Geometry: final body of the model. Coordinates: model frame, mm. A direction names the side the tool comes from. Give positions to 0.01 mm unless a question says otherwise; leave off trailing zeros. Write each loop counter-clockwise with the first axis right and the second up, starting at its lowest first coordinate (ties: lowest second). Pieces come first, ordered by that corner, then holes.
from build123d import *

# Parameters (mm, degrees)
SKETCH1_W                = 80
SKETCH1_H                = 80
BOSS_EXTRUDE1_DEPTH      = 2
SKETCH2_W                = 80
SKETCH2_H                = 2
BOSS_EXTRUDE2_DEPTH      = 50
SKETCH3_W                = 2
SKETCH3_H                = 76
BOSS_EXTRUDE3_DEPTH      = 50
CUT_EXTRUDE2_DEPTH       = 100
SKETCH6_W                = 2
SKETCH6_H                = 76
BOSS_EXTRUDE4_DEPTH      = 16.666666667
BOSS_EXTRUDE5_DEPTH      = 2
BOSS_EXTRUDE5_DEPTH_BACK = 82
SKETCH7_W                = 84
SKETCH7_H                = 9.392000317
SKETCH8_W                = 14
SKETCH8_H                = 80
CUT_EXTRUDE3_DEPTH       = 50


with BuildPart() as part:
    # Sketch1 → Boss-Extrude1 (new body)
    with BuildSketch(Plane.XY):
        with Locations((40, 40)):
            Rectangle(SKETCH1_W, SKETCH1_H)
    extrude(amount=BOSS_EXTRUDE1_DEPTH)

    # Sketch2 → Boss-Extrude2 (add)
    with BuildSketch(Plane(origin=(0, 0, 0), x_dir=(-1, 0, 0), z_dir=(0, 0, -1))):
        with Locations((-40, 79)):
            Rectangle(SKETCH2_W, SKETCH2_H)
        with Locations((-40, 1)):
            Rectangle(SKETCH2_W, SKETCH2_H)
    extrude(amount=BOSS_EXTRUDE2_DEPTH)

    # Sketch3 → Boss-Extrude3 (add)
    with BuildSketch(Plane(origin=(0, 0, 0), x_dir=(-1, 0, 0), z_dir=(0, 0, -1))):
        with Locations((-79, 40)):
            Rectangle(SKETCH3_W, SKETCH3_H)
    extrude(amount=BOSS_EXTRUDE3_DEPTH)

    # Sketch5 → Cut-Extrude2 (cut)
    with BuildSketch(Plane(origin=(0, 80, 0), x_dir=(1, 0, 0), z_dir=(0, 1, 0))):
        Polygon((80, 50), (0, 16.666666667), (0, 50), align=None)
    extrude(amount=-CUT_EXTRUDE2_DEPTH, mode=Mode.SUBTRACT)

    # Sketch6 → Boss-Extrude4 (add)
    with BuildSketch(Plane(origin=(0, 0, 0), x_dir=(-1, 0, 0), z_dir=(0, 0, -1))):
        with Locations((-1, 40)):
            Rectangle(SKETCH6_W, SKETCH6_H)
    extrude(amount=BOSS_EXTRUDE4_DEPTH)

    # Sketch7 → Boss-Extrude5 (add, two sides: drawn at the far end of the back side and taken through both)
    with BuildSketch(Plane(origin=(0, 80, 0), x_dir=(1, 0, 0), z_dir=(0, 1, 0)).offset(-BOSS_EXTRUDE5_DEPTH_BACK)):
        with Locations((52, 7.482577596)):
            Rectangle(SKETCH7_W, SKETCH7_H)
    extrude(amount=BOSS_EXTRUDE5_DEPTH + BOSS_EXTRUDE5_DEPTH_BACK)

    # Sketch8 → Cut-Extrude3 (cut)
    with BuildSketch(Plane.XY.offset(-2.786577437)):
        with Locations((87, 40)):
            Rectangle(SKETCH8_W, SKETCH8_H)
    extrude(amount=-CUT_EXTRUDE3_DEPTH, mode=Mode.SUBTRACT)


solid = part.part
Q1. Section C-C on y = 35. Output: boundary loops of the cut face in (x, z), plus the area to 3 significant figures.
Filled sheet:
outline: (0, -16.67) - (2, -16.67) - (2, 0) - (78, 0) - (78, -2.79) - (10, -2.79) - (10, -12.18) - (78, -12.18) - (78, -49.17) - (80, -50) - (80, 2) - (0, 2) - close
area: 931 mm2
Q2. Section D-D on x = 58. Output: boundary loops of the cut face in (y, z).
Filled sheet:
outline: (-2, -12.18) - (0, -12.18) - (0, -40.83) - (2, -40.83) - (2, -12.18) - (78, -12.18) - (78, -40.83) - (80, -40.83) - (80, -12.18) - (82, -12.18) - (82, -2.79) - (80, -2.79) - (80, 2) - (0, 2) - (0, -2.79) - (-2, -2.79) - close; hole (2, -2.79) - (78, -2.79) - (78, 0) - (2, 0) - close
Q3. Pull-direction query (X, two-part tool) for faces 5 (the flat face through (80, 39, -24)), 6 (the flat face through (39, 41, 0)), 7 (the flat face through (0, 39, -7)), 8 (the flat face through (39, 41, 2)); classes: released by +X, released by -X, zero draft, split by the parting line, or undercut.
Filled sheet:
face 5: released by +X
face 6: undercut
face 7: released by -X
face 8: zero draft
Q4. Section B-B on z = -43. Output: boundary loops of the cut face in (x, y).
Filled sheet:
outline: (63.2, 0) - (80, 0) - (80, 80) - (63.2, 80) - (63.2, 78) - (78, 78) - (78, 2) - (63.2, 2) - close
Q5. Section A-A on x = 88. Output: boundary loops of the cut face in (y, z).
Filled sheet:
outline: (-2, -12.18) - (0, -12.18) - (0, -2.79) - (-2, -2.79) - close; (80, -12.18) - (82, -12.18) - (82, -2.79) - (80, -2.79) - close
Q6. Pin query (flat end, axial travel): P1, Ø0.6, axis at x = 65, y = -1.5, coming from the +Z side; P2, Ø10, axis at y = 23, z = -24.5, coming from the +X side; P3, Ø10, axis at x = 54.5, z = -30.5, coming from the -Y side. Return the tip coordinate at first contact, or that it passes through.
Filled sheet:
P1: stops at z = -2.79
P2: stops at x = 80
P3: stops at y = 0
Q7. Ray query, line 1 along X through (y, z) = (56, -13); line 2 along Z through (x, y) = (61, 36). Return the intervals inside material, ascending.
Filled sheet:
line 1: x = 0 to 2, 78 to 80
line 2: z = -12.18 to -2.79, 0 to 2
Q8. Access query for faces 1 (the flat face through (87, 0, -7)), 2 (the flat face through (48, 78, -19)), 3 (the flat face through (51, -2, -8)), 4 (the flat face through (10, 39, -7)). Directions: +Z, -Z, +X, -X, +Y, -Y. A direction counts if a zero-diameter tool reaches every point of the face in a straight line with its end or side. Return the directions, or none.
Filled sheet:
face 1: +Z, -Z, +X
face 2: none
face 3: +Z, -Z, +X, -X, -Y
face 4: -Z
